```python
from build123d import *

# Parameters (mm, degrees)
SKETCH1_R           = 25
BOSS_EXTRUDE1_DEPTH = 2
SKETCH1_3_R         = 23.5
BOSS_EXTRUDE2_DEPTH = 1
CUT_EXTRUDE1_REACH  = 4
SKETCH1_4_R         = 22.5
SKETCH1_5_R         = 22.5
BOSS_EXTRUDE3_DEPTH = 0.5
SKETCH2_R           = 2.398519327
CUT_EXTRUDE2_DEPTH  = 10.5
CIRPATTERN1_COUNT   = 4


with BuildPart() as part:
    # Sketch1 → Boss-Extrude1 (new body)
    with BuildSketch(Plane.XY):
        Circle(SKETCH1_R)
    extrude(amount=BOSS_EXTRUDE1_DEPTH)

    # Sketch1_3 → Boss-Extrude2 (add)
    with BuildSketch(Plane.XY):
        Circle(SKETCH1_3_R)
    extrude(amount=-BOSS_EXTRUDE2_DEPTH)

    # Sketch1_4 → Cut-Extrude1 (cut, up to next)
    with BuildSketch(Plane.XY, mode=Mode.PRIVATE) as cut_extrude1_sk1:
        Circle(SKETCH1_4_R)
    cut_extrude1_tool1 = extrude(cut_extrude1_sk1.sketch, amount=CUT_EXTRUDE1_REACH, mode=Mode.PRIVATE) & part.part
    add(cut_extrude1_tool1.solids().sort_by_distance((0, 0, 0))[0], mode=Mode.SUBTRACT)

    # Sketch1_5 → Boss-Extrude3 (add)
    with BuildSketch(Plane.XY):
        Circle(SKETCH1_5_R)
    extrude(amount=BOSS_EXTRUDE3_DEPTH)

    # Sketch2 → Cut-Extrude2 (cut)
    with BuildSketch(Plane(origin=(0, 0, -1), x_dir=(-1, 0, 0), z_dir=(0, 0, -1))):
        with Locations((12.727922061, 12.727922061)):
            Circle(SKETCH2_R)
    cut_extrude2 = extrude(amount=-CUT_EXTRUDE2_DEPTH, mode=Mode.SUBTRACT)

    # CirPattern1: Cut-Extrude2 ×4 about axis
    cirpattern1_axis = Axis((0, 0, 0), (0, 0, 1))
    for i in range(1, CIRPATTERN1_COUNT):
        add(cut_extrude2.rotate(cirpattern1_axis, i * 360 / CIRPATTERN1_COUNT), mode=Mode.SUBTRACT)


solid = part.part
```
The listing builds one solid part. Answer for the finished solid, in the listing's coordinates (mm). A direction names the side the tool comes from. Give positions to 0.01 mm unless a question says otherwise; leave off trailing zeros. Order: outer loops, then holes, each group sorted by start corner. A loop starts at its lowest first (then second) coordinate and runs counter-clockwise, first axis right, second up. Notation, with made-up numbers: (78, 32.5) - (121, 32.5) arc R26 cw to (121, 62.5) - close; hole circle Ø1 at (22, 5.25). An arc over 180 degrees is marked (long way). Use one line per item in the form item = value. Start each with the question number.
(1) For faces 1 (the cylindrical face through (22.4, 7.1, -0.5)), 2 (the cylindrical face through (10.382, -19.961, 1.24)), 3 (the flat face through (-22.34, 3.82, 2)), determine the directions among +Z, -Z, +X, -X, +Y, -Y from which every point of the face is accessible in a straight line to the end or side of a thin tool.
(2) A cutting plane is placed at B-B, the plane y = -11.5. Write down the section's boundary in (x, z), then the cut area to 3 significant figures.
(3) Flat-ended cylindrical pins translate along their axes: pin 1 Ø1.5 at (x, y) = (-12.5, -6.5) entering from +Z; pin 2 Ø4 at (x, y) = (12.73, -12.73) entering from +Z. Find the tip coordinate at first contact, or state that the pin passes through.
(4) Consider line 1 (Y direction, x = -12, z = 0.4); line 2 (Y direction, x = -12, z = -0.65); line 3 (Z direction, x = -6.5, y = -14). Determine where each line is inside the solid, lowest interval first. Write a range as from..to.
(5) A cutting plane is placed at A-A, the plane x = 0. Write down the section's boundary in (y, z).
(6) The mould has two halves that part along X. Classify faces 4 (the cylindrical face through (23.846, 7.509, 0.986)), 5 (the flat face through (0, 0, -1)), 6 (the flat face through (0, 0, 0.5)): released by +X, released by -X, zero draft, split by the parting line, or undercut.
(7) A cutting plane is placed at D-D, the plane x = -13.5. Write down the section's boundary in (y, z).
Ans:
q1.face_1 = -Z
q1.face_2 = +Z
q1.face_3 = +Z, +X, -X, +Y, -Y
q2.outline = (-22.2, 0) - (-20.49, 0) - (-20.49, -1) - (-14.79, -1) - (-14.79, 0.5) - (-19.34, 0.5) - (-19.34, 2) - (-22.2, 2) - close; (-10.67, -1) - (10.67, -1) - (10.67, 0.5) - (-10.67, 0.5) - close; (14.79, -1) - (20.49, -1) - (20.49, 0) - (22.2, 0) - (22.2, 2) - (19.34, 2) - (19.34, 0.5) - (14.79, 0.5) - close
q2.area = 59.4 mm^2
q3.pin_1 = 0.5
q3.pin_2 = through
q4.line_1 = -21.93..-15.01, -10.44..10.44, 15.01..21.93
q4.line_2 = -20.21..-15.01, -10.44..10.44, 15.01..20.21
q4.line_3 = -1..0.5
q5.outline = (-25, 0) - (-23.5, 0) - (-23.5, -1) - (23.5, -1) - (23.5, 0) - (25, 0) - (25, 2) - (22.5, 2) - (22.5, 0.5) - (-22.5, 0.5) - (-22.5, 2) - (-25, 2) - close
q6.face_4 = split by the parting line
q6.face_5 = zero draft
q6.face_6 = undercut
q7.outline = (-21.04, 0) - (-19.24, 0) - (-19.24, -1) - (-15, -1) - (-15, 0.5) - (-18, 0.5) - (-18, 2) - (-21.04, 2) - close; (-10.46, -1) - (10.46, -1) - (10.46, 0.5) - (-10.46, 0.5) - close; (15, -1) - (19.24, -1) - (19.24, 0) - (21.04, 0) - (21.04, 2) - (18, 2) - (18, 0.5) - (15, 0.5) - close
